CAD build for the part. Positions are in the model's coordinates, mm. Face numbers are marked on the shaded views. A direction names the side the tool comes from. Round coordinates to 2 decimals unless told otherwise and drop trailing zeros. Loops run counter-clockwise (first coordinate to the right, second up) from the corner with the lowest first, then second, coordinate; pieces in that order, holes last. Notation, with made-up numbers: (55.5, 72) - (76.5, 72) arc R17 cw to (76.5, 98) - close; hole circle Ø7 at (58, 88). An arc over 180 degrees is marked (long way). Use one line per item in the form item = value.
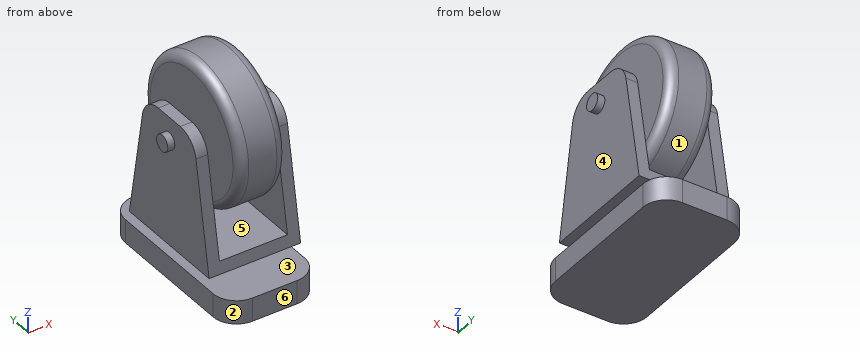
from build123d import *

# Parameters (mm, degrees)
SKETCH1_W           = 39
SKETCH1_H           = 75
BOSS_EXTRUDE1_DEPTH = 10
SKETCH2_R           = 10
BOSS_EXTRUDE2_DEPTH = 5
SKETCH3_W           = 39
SKETCH3_H           = 50
BOSS_EXTRUDE3_DEPTH = 5
SKETCH4_W           = 5
SKETCH4_H           = 50
BOSS_EXTRUDE4_DEPTH = 50
CUT_EXTRUDE1_REACH  = 830.882
FILLET1_R           = 10
SKETCH6_R           = 30
BOSS_EXTRUDE5_DEPTH = 10
SKETCH7_R           = 3.5
BOSS_EXTRUDE6_DEPTH = 22.5
FILLET2_R           = 4
FILLET3_R           = 10


with BuildPart() as part:
    # Sketch1 → Boss-Extrude1 (new body)
    with BuildSketch(Plane.XY):
        with Locations((-295.5, 787.5)):
            Rectangle(SKETCH1_W, SKETCH1_H)
    extrude(amount=BOSS_EXTRUDE1_DEPTH)

    # Sketch2 → Boss-Extrude2 (add)
    with BuildSketch(Plane.XY.offset(10)):
        with Locations(Location((-295.5, 787.5, 0), (0, 0, 180))):
            Circle(SKETCH2_R)
    extrude(amount=BOSS_EXTRUDE2_DEPTH)

    # Sketch3 → Boss-Extrude3 (add)
    with BuildSketch(Plane.XY.offset(15)):
        with Locations((-295.5, 787.5)):
            Rectangle(SKETCH3_W, SKETCH3_H)
    extrude(amount=BOSS_EXTRUDE3_DEPTH)

    # Sketch4 → Boss-Extrude4 (add)
    with BuildSketch(Plane.XY.offset(20)):
        with Locations((-278.5, 787.5)):
            Rectangle(SKETCH4_W, SKETCH4_H)
        with Locations((-312.5, 787.5)):
            Rectangle(SKETCH4_W, SKETCH4_H)
    extrude(amount=BOSS_EXTRUDE4_DEPTH)

    # Cut-Extrude1: up to this face of the body (flat: up to its plane)
    cut_extrude1_end = Plane(part.part.faces().sort_by_distance((-315, 787.5, 42.5))[0])
    # Sketch5 → Cut-Extrude1 (cut, up to the picked face)
    with BuildSketch(Plane(origin=(-276, 0, 0), x_dir=(0, 0, -1), z_dir=(1, 0, 0)), mode=Mode.PRIVATE) as cut_extrude1_sk1:
        Polygon((-15, 812.5), (-70, 802.802016061), (-70, 812.5), align=None)
    cut_extrude1_tool1 = split(extrude(cut_extrude1_sk1.sketch, amount=-CUT_EXTRUDE1_REACH, mode=Mode.PRIVATE), bisect_by=cut_extrude1_end, keep=Keep.BOTH, mode=Mode.PRIVATE)
    # Sketch5 → Cut-Extrude1 (cut, up to the picked face)
    with BuildSketch(Plane(origin=(-276, 0, 0), x_dir=(0, 0, -1), z_dir=(1, 0, 0)), mode=Mode.PRIVATE) as cut_extrude1_sk2:
        Polygon((-70, 762.5), (-15, 762.5), (-70, 772.197983939), align=None)
    cut_extrude1_tool2 = split(extrude(cut_extrude1_sk2.sketch, amount=-CUT_EXTRUDE1_REACH, mode=Mode.PRIVATE), bisect_by=cut_extrude1_end, keep=Keep.BOTH, mode=Mode.PRIVATE)
    add(cut_extrude1_tool1.solids().sort_by(Axis((-276, 809.267339, 51.666667), (-1, 0, 0)))[0], mode=Mode.SUBTRACT)
    add(cut_extrude1_tool2.solids().sort_by(Axis((-276, 765.732661, 51.666667), (-1, 0, 0)))[0], mode=Mode.SUBTRACT)

    # Fillet1
    fillet1_edges = [part.edges().sort_by_distance(p)[0] for p in [
        (-315, 825, 5),
        (-276, 825, 5),
        (-276, 750, 5),
        (-315, 750, 5),
    ]]
    fillet(fillet1_edges, radius=FILLET1_R)



with BuildPart() as body_2:
    # Sketch6 → Boss-Extrude5 (new, symmetric)
    with BuildSketch(Plane(origin=(-295.5, 0, 0), x_dir=(0, 0, -1), z_dir=(1, 0, 0))):
        with Locations((-60, 787.5)):
            Circle(SKETCH6_R)
    extrude(amount=BOSS_EXTRUDE5_DEPTH, both=True)


with BuildPart() as part_1:
    add(part.part)

    add(body_2.part)  # Boss-Extrude6 merges body 2
    # Sketch7 → Boss-Extrude6 (add, symmetric)
    with BuildSketch(Plane(origin=(-295.5, 0, 0), x_dir=(0, 0, -1), z_dir=(1, 0, 0))):
        with Locations(Location((-60, 787.5, 0), (0, 0, 180))):
            Circle(SKETCH7_R)
    extrude(amount=BOSS_EXTRUDE6_DEPTH, both=True)

    # Fillet2
    fillet2_edges = [part_1.edges().sort_by_distance(p)[0] for p in [
        (-305.5, 787.5, 90),
        (-285.5, 787.5, 90),
    ]]
    fillet(fillet2_edges, radius=FILLET2_R)

    # Fillet3
    fillet3_edges = [part_1.edges().sort_by_distance(p)[0] for p in [
        (-278.5, 802.802016061, 70),
        (-312.5, 802.802016061, 70),
        (-278.5, 772.197983939, 70),
        (-312.5, 772.197983939, 70),
    ]]
    fillet(fillet3_edges, radius=FILLET3_R)


solid = part_1.part
1) Drill centre lines: probe 1 along X at (y, z) = (785, 49.5); probe 2 along Z at (x, y) = (-306, 803); probe 3 along Z at (x, y) = (-286, 771). Where is each one in solid material? Low to high.
Report:
probe_1 = -315 to -310, -305.5 to -285.5, -281 to -276
probe_2 = 0 to 10, 15 to 20
probe_3 = 0 to 10, 15 to 20, 37.46 to 82.54
2) Slice it at D-D (y = 768). State how many separate pieces and enclosed holes the cut face has, plus the area to 3 significant figures.
Report:
separate_pieces = 3
enclosed_holes = 0
area = 1,740 mm^2
3) Tool access for the marked faces 5 and 6: list every direction of +Z, -Z, +X, -X, +Y, -Y with a clear straight run to the whole face (end or side of a thin tool).
Report:
face_5 = +Y, -Y
face_6 = +Z, -Z, +X, -X, -Y
4) Slice it at B-B (x = -308). Write the cut outline in (y, z).
Report:
outline = (750.46, 0) - (824.54, 0) - (824.54, 10) - (750.46, 10) - close; (762.5, 15) - (812.5, 15) - (811.62, 20) - (763.38, 20) - close; circle Ø7 at (787.5, 60)
5) Two-plate mould, pull along X, no slides. Class the marked faces 1, 2, 3 and 4: +X half, -X half, draft (parallel to the pull), parting line (faces both ways), or undercut.
Report:
face_1 = undercut
face_2 = -X half
face_3 = draft
face_4 = +X half
6) Slice it at C-C (z = 6.5). Write the cut outline in (x, y).
Report:
outline = (-315, 760) arc R10 ccw to (-305, 750) - (-286, 750) arc R10 ccw to (-276, 760) - (-276, 815) arc R10 ccw to (-286, 825) - (-305, 825) arc R10 ccw to (-315, 815) - close
7) Slice it at A-A (x = -295.5). Write the cut outline in (y, z), plus the area to 3 significant figures.
Report:
outline = (750, 0) - (825, 0) - (825, 10) - (797.5, 10) - (797.5, 15) - (812.5, 15) - (811.62, 20) - (763.38, 20) - (762.5, 15) - (777.5, 15) - (777.5, 10) - (750, 10) - close; circle Ø60 at (787.5, 60)
area = 3,920 mm^2
8) Flat gauge pins, fed straight in: pin 1 (5 mm diameter, centred on y = 777.5, z = 6.5, fed in from +X); pin 2 (5.5 mm diameter, centred on x = -312, y = 787.5, fed in from +Z); pin 3 (11.5 mm diameter, centred on x = -286.5, y = 798.5, fed in from +Z); pin 4 (3 mm diameter, centred on y = 814, z = 20, fed in from -X). Where does each tip first touch, or does it go through?
Report:
pin_1 = -276
pin_2 = 70
pin_3 = 89.4
pin_4 = through
